CAD build for the part. Positions are in the model's coordinates, mm. A direction names the side the tool comes from. Coordinates: 2 decimals unless noted, no trailing zeros. Loops run counter-clockwise (first coordinate to the right, second up) from the corner with the lowest first, then second, coordinate; pieces in that order, holes last. Notation, with made-up numbers: (79, 49) -> (103, 49) arc R25 cw to (103, 83) -> close; hole circle Ø2 at (5, 12). An arc over 180 degrees is marked (long way). Return JSON: item names as keys, results as strings. Group by question number.
(1) Flat gauge pins, fed straight in: pin 1 Ø1.5 at (y, z) = (2, 2) entering from -X; pin 2 Ø0.9 at (y, z) = (54.5, 1.5) entering from -X; pin 3 Ø0.9 at (y, z) = (1.5, 1) entering from +X. Where does each tip first touch, or does it go through?
(2) Tool access for faces 1 (the face through (6, 3, 2)), 2 (the face through (11, 52.5, 2)), 3 (the face through (18, 1, 2)), 4 (the face through (3, 27, 2)): list every direction of +Z, -Z, +X, -X, +Y, -Y with a clear straight run to the whole face (end or side of a thin tool).
(3) Saw through at A-A on z = 2.3. Write the cut outline in (x, y).
(4) Saw through at B-B on x = 8.5. Write the cut outline in (y, z), then the cut area to 4 significant figures.
(5) Probe L1, parallel to Y at x = 18.25, z = 1.85; L2, parallel to Y at x = 15, z = 0.4. List the from-to ranges inside material, lowest first.
Autodesk Inventor part; units mm, degrees
ref_plane "YZ Plane" through (0, 0, 0) normal (1, 0, 0) x (0, 1, 0)
ref_plane "XZ Plane" through (0, 0, 0) normal (0, 1, 0) x (-1, 0, 0)
ref_plane "XY Plane" through (0, 0, 0) normal (0, 0, 1) x (1, 0, 0)
sketch "Sketch1" plane through (0, 0, 0) normal (0, 0, 1) x (1, 0, 0)
  line L0 (0, 0) -> (25, 0)
  line L1 (25, 0) -> (25, 55.5)
  line L2 (25, 55.5) -> (0, 55.5)
  line L3 (0, 55.5) -> (0, 0)
  dimension "d0" = 25
  dimension "d1" = 55.5
extrude "Extrusion1" add sketch "Sketch1" along normal blind 3
sketch "Sketch2" plane through (0, 0, 3) normal (0, 0, 1) x (1, 0, 0)
  line L0 (0, 55.5) -> (0, 0)
  line L1 (25, 55.5) -> (0, 55.5)
  line L2 (0, 0) -> (3, 0)
  line L3 (3, 0) -> (3, 55.5)
  line L4 (3, 55.5) -> (0, 55.5)
  line L5 (0, 55.5) -> (0, 0)
  dimension "d4" = 3
extrude "Extrusion2" cut sketch "Sketch2" against normal through all
sketch "Sketch3" plane through (0, 0, 3) normal (0, 0, 1) x (1, 0, 0)
  point P0 (0, 0)
sketch "Sketch4" plane through (0, 0, 3) normal (0, 0, 1) x (1, 0, 0)
  line L0 (25, 55.5) -> (3, 55.5)
  line L1 (3, 55.5) -> (18.5, 55.5)
  line L2 (18.5, 55.5) -> (18.5, 22.5)
  line L3 (18.5, 22.5) -> (3, 22.5)
  line L4 (3, 22.5) -> (3, 55.5)
  point P0 (0, 0)
  dimension "d7" = 15.5
  dimension "d8" = 33
sketch "Sketch5" plane through (0, 0, 3) normal (0, 0, 1) x (1, 0, 0)
  line L0 (3, 0) -> (25, 0)
  line L1 (8, 0) -> (18, 0)
  line L2 (18, 0) -> (18, 3)
  line L3 (18, 3) -> (8, 3)
  line L4 (8, 3) -> (8, 0)
  line L5 (3, 55.5) -> (3, 0)
  line L6 (3, 0) -> (8, 0)
  line L7 (8, 0) -> (8, 3)
  line L8 (8, 3) -> (3, 3)
  line L9 (3, 3) -> (3, 0)
  line L10 (18, 0) -> (25, 0)
  line L11 (25, 0) -> (25, 3)
  line L12 (25, 3) -> (18, 3)
  line L13 (18, 3) -> (18, 0)
  point P0 (0, 0)
  point P1 (3, 22.5)
  dimension "d11" = 10
  dimension "d12" = 3
  dimension "d13" = 5
extrude "Extrusion4" cut sketch "Sketch5" against normal through all contours L5 L8 L4 L0 | L2 L12 L11 L0
sketch "Sketch6" plane through (0, 0, 3) normal (0, 0, 1) x (1, 0, 0)
  line L0 (25, 55.5) -> (3, 55.5)
  line L1 (3, 55.5) -> (18.5, 55.5)
  line L2 (18.5, 55.5) -> (18.5, 52.5)
  line L3 (18.5, 52.5) -> (3, 52.5)
  line L4 (3, 52.5) -> (3, 55.5)
  line L5 (18.5, 55.5) -> (18.5, 22.5)
  point P0 (0, 0)
  dimension "d16" = 3
extrude "Extrusion5" cut sketch "Sketch6" against normal through all
properties part number "hollow_mount"
Geometry results:
{
 "1": {"pin 1": "x = 8", "pin 2": "x = 18.5", "pin 3": "x = 18"},
 "2": {"face 1": "+Z, -Z, -X, -Y", "face 2": "+Z, -Z, -X, +Y", "face 3": "+Z, -Z, +X, -Y", "face 4": "+Z, -Z, -X, +Y, -Y"},
 "3": {"outline": "(3, 3) -> (8, 3) -> (8, 0) -> (18, 0) -> (18, 3) -> (25, 3) -> (25, 55.5) -> (18.5, 55.5) -> (18.5, 52.5) -> (3, 52.5) -> close"},
 "4": {"outline": "(0, 0) -> (52.5, 0) -> (52.5, 3) -> (0, 3) -> close", "area": "157.5 mm²"},
 "5": {"L1": "3 to 52.5", "L2": "0 to 52.5"}
}
